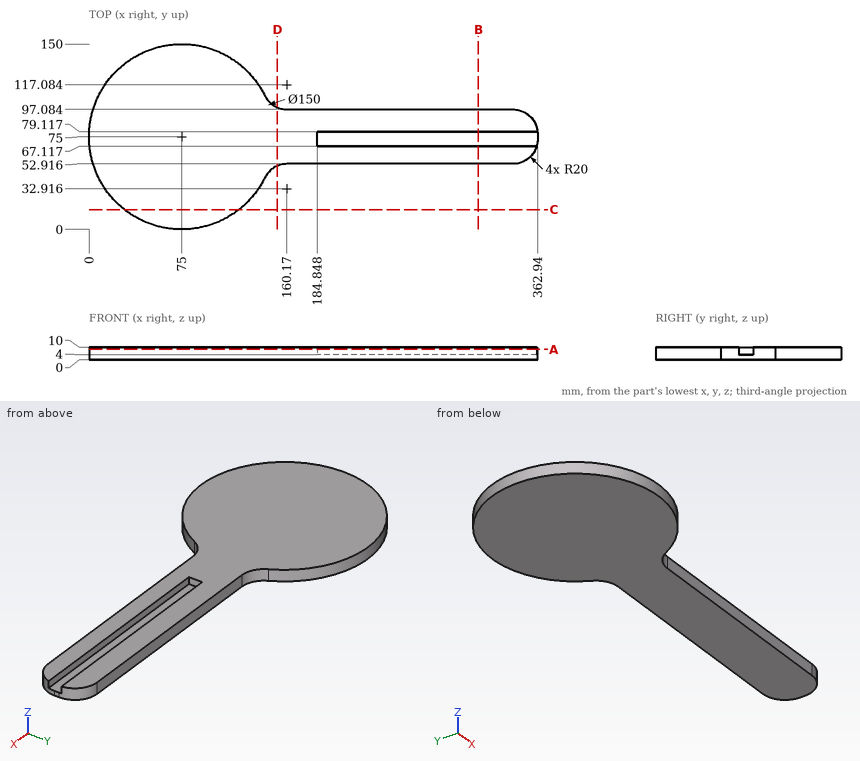
Check sheet for the drawn part. Datum: minimum x, y, z corner. Units: mm. Give positions to 0.01 mm unless a question says otherwise; leave off trailing zeros. Loops run counter-clockwise (first coordinate to the right, second up) from the corner with the lowest first, then second, coordinate; pieces in that order, holes last.
1) Sectioned sample at A-A, the plane z = 8.5. Enter the section's corners in (x, y).
2) Thickness scan on line 1 along Y through (x, z) = (319.5, 6.25); line 2 along Y through (x, z) = (159, 8); line 3 along Z through (x, y) = (288, 76). Record the ranges inside material, lowest first.
3) Sectioned sample at B-B, the plane x = 315. Enter the section's corners in (y, z), then the cut area to 3 significant figures.
4) Sectioned sample at C-C, the plane y = 16. Enter the section's corners in (x, z), then the cut area to 3 significant figures.
5) Sectioned sample at D-D, the plane x = 152.5. Enter the section's corners in (y, z), then the cut area to 3 significant figures.
6) Depth check by flat-ended pin: pin 1 Ø3 at (x, z) = (95.5, 4.5) entering from +Y; pin 2 Ø1 at (x, z) = (295, 2) entering from +Y; pin 3 Ø3 at (y, z) = (132, 1) entering from -X (1 decimal); pin 4 Ø6 at (x, y) = (124.5, 89.5) entering from -Z. Enter the tip coordinate at first touch or a pass-through.
Answers:
1. outline: (142.24, 41.78) arc R20 cw to (160.17, 52.92) - (342.94, 52.92) arc R20 ccw to (362.08, 67.12) - (184.85, 67.12) - (184.85, 79.12) - (362.84, 79.12) arc R20 ccw to (342.94, 97.08) - (160.17, 97.08) arc R20 cw to (142.24, 108.22) arc R75 ccw (long way) to start
2. line 1: y = 52.92 to 67.12, 79.12 to 97.08
2. line 2: y = 52.88 to 97.12
2. line 3: z = 0 to 4
3. outline: (52.92, 0) - (97.08, 0) - (97.08, 10) - (79.12, 10) - (79.12, 4) - (67.12, 4) - (67.12, 10) - (52.92, 10) - close
3. area: 370 mm2
4. outline: (28.7, 0) - (121.3, 0) - (121.3, 10) - (28.7, 10) - close
4. area: 926 mm2
5. outline: (51.39, 0) - (98.61, 0) - (98.61, 10) - (51.39, 10) - close
5. area: 472 mm2
6. pin 1: stops at y = 147.55
6. pin 2: stops at y = 97.08
6. pin 3: stops at x = 24.6
6. pin 4: stops at z = 0
